Geometry: final body of the model. Coordinates: model frame, mm. A direction names the side the tool comes from. Give positions to 0.01 mm unless a question says otherwise; leave off trailing zeros. Write each loop counter-clockwise with the first axis right and the second up, starting at its lowest first coordinate (ties: lowest second). Pieces come first, ordered by that corner, then holes. Notation, with made-up numbers: M 20.25,12 L 78.25,12 A34 ccw 78.25,42 Z; hole C 72.5,33.5 d1. An arc over 180 degrees is marked long. One line per question, with ' | ' between items.
from build123d import *

# Parameters (mm, degrees)
BOSS_EXTRUDE1_DEPTH = 6.35
SKETCH2_R           = 1.524
CUT_EXTRUDE1_DEPTH  = 7.35


with BuildPart() as part:
    # Sketch1 → Boss-Extrude1 (new body)
    with BuildSketch(Plane.XY):
        Polygon((50.8, 25.4), (0, 25.4), (0, 6.35), (4.826, 6.35), (4.826, 10.414), (3.048, 10.414), (3.048, 12.7), (4.826, 12.7), (4.826, 16.51), (7.874, 16.51), (7.874, 12.7), (9.652, 12.7), (9.652, 10.414), (7.874, 10.414), (7.874, 6.35), (12.7, 6.35), (12.7, 0), (38.1, 0), (38.1, 6.35), (42.926, 6.35), (42.926, 10.414), (41.148, 10.414), (41.148, 12.7), (42.926, 12.7), (42.926, 16.51), (45.974, 16.51), (45.974, 12.7), (47.752, 12.7), (47.752, 10.414), (45.974, 10.414), (45.974, 6.35), (50.8, 6.35), align=None)
    extrude(amount=BOSS_EXTRUDE1_DEPTH)

    # Sketch2 → Cut-Extrude1 (cut, through all)
    with BuildSketch(Plane.XY.offset(6.35)):
        with Locations((25.4, 20.32)):
            Circle(SKETCH2_R)
    extrude(amount=-CUT_EXTRUDE1_DEPTH, mode=Mode.SUBTRACT)


solid = part.part
(1) First-contact query: P1, Ø1.5, axis at x = 6.5, z = 2.5, coming from the -Y side; P2, Ø1.4, axis at x = 10, z = 1.5, coming from the -Y side; P3, Ø1.8, axis at x = 25.4, y = 20.32, coming from the +Z side. Flat tips, straight axial feed; report the tip coordinate or a pass-through.
Working result:
P1: stops at y = 16.51 | P2: stops at y = 6.35 | P3: passes through
(2) Cut plane B-B, the plane x = 25.4. Return loops of the section in (y, z).
Working result:
outline: M 0,0 L 18.8,0 L 18.8,6.35 L 0,6.35 Z; M 21.84,0 L 25.4,0 L 25.4,6.35 L 21.84,6.35 Z
(3) Cut plane A-A, the plane y = 15.75. Return loops of the section in (x, z), then the cut area to 3 significant figures.
Working result:
outline: M 0,0 L 4.83,0 L 4.83,6.35 L 0,6.35 Z; M 7.87,0 L 42.93,0 L 42.93,6.35 L 7.87,6.35 Z; M 45.97,0 L 50.8,0 L 50.8,6.35 L 45.97,6.35 Z | area: 284 mm^2
(4) Draft query along X for faces 4 (the face through (4, 12.7, 3)), 5 (the face through (25, 13, 6.35)), 6 (the face through (0, 16, 3)). Return one class per face: released by +X, released by -X, zero draft, split by the parting line, or undercut.
Working result:
face 4: undercut | face 5: zero draft | face 6: released by -X
(5) Set-up query: faces 1 (the face through (42, 10.414, 3)), 2 (the face through (10, 6.35, 3)), 3 (the face through (45.974, 15, 3)). Return all of +Z, -Z, +X, -X, +Y, -Y with unobstructed straight access to the full face (end or side cutting, diameter ignored); none if empty.
Working result:
face 1: +Z, -Z | face 2: +Z, -Z, -X, -Y | face 3: +Z, -Z, -Y
(6) Material intervals for L1, parallel to X at y = 6.5, z = 1.5; L2, parallel to Y at x = 9.5, z = 6; L3, parallel to Y at x = 25.4, z = 4.75, sorted ascending. Write a range as [from, to].
Working result:
L1: x = [0, 4.83], [7.87, 42.93], [45.97, 50.8] | L2: y = [6.35, 10.41], [12.7, 25.4] | L3: y = [0, 18.8], [21.84, 25.4]
(7) Cut plane C-C, the plane y = 20.32. Return loops of the section in (x, z), then the cut area to 3 significant figures.
Working result:
outline: M 0,0 L 23.88,0 L 23.88,6.35 L 0,6.35 Z; M 26.92,0 L 50.8,0 L 50.8,6.35 L 26.92,6.35 Z | area: 303 mm^2
